```python
from build123d import *

# Parameters (mm, degrees)
CYLINDER038_R     = 0.8
CYLINDER038_DEPTH = 30
BOX040_W          = 21
BOX040_H          = 20
BOX040_DEPTH      = 18
CHAMFER_SIZE      = 8
BOX041_W          = 13
BOX041_H          = 20
BOX041_DEPTH      = 5
FILLET002033_R    = 3
BOX031_W          = 21
BOX031_H          = 20
BOX031_DEPTH      = 18
FILLET002030_R    = 3
FILLET002031_R    = 3
FILLET002032_R    = 3


with BuildPart() as obj1:
    # Cylinder038 → Cylinder038 (new body)
    with BuildSketch(Plane(origin=(42, 45, 26), x_dir=(1, 0, 0), z_dir=(0, 1, 0))):
        Circle(CYLINDER038_R)
    extrude(amount=CYLINDER038_DEPTH)


with BuildPart() as fusion024:
    # Box040 → Box040 (new body)
    with BuildSketch(Plane(origin=(40, 51.5, 10), x_dir=(1, 0, 0), z_dir=(0, 0, 1))):
        with Locations((10.5, 10)):
            Rectangle(BOX040_W, BOX040_H)
    extrude(amount=BOX040_DEPTH)

    # Chamfer
    chamfer_edges = [fusion024.edges().sort_by_distance(p)[0] for p in [
        (40, 61.5, 28),
    ]]
    chamfer(chamfer_edges, length=CHAMFER_SIZE)

    # Fusion024: union obj1
    add(obj1.part)


with BuildPart() as fillet002033:
    # Box041 → Box041 (new body)
    with BuildSketch(Plane(origin=(45, 51.5, 28), x_dir=(1, 0, 0), z_dir=(0, 0, 1))):
        with Locations((6.5, 10)):
            Rectangle(BOX041_W, BOX041_H)
    extrude(amount=BOX041_DEPTH)

    # Fillet002033
    fillet002033_edges = [fillet002033.edges().sort_by_distance(p)[0] for p in [
        (45, 51.5, 30.5),
        (45, 71.5, 30.5),
        (58, 51.5, 30.5),
        (58, 71.5, 30.5),
    ]]
    fillet(fillet002033_edges, radius=FILLET002033_R)


with BuildPart() as button:
    # Box031 → Box031 (new body)
    with BuildSketch(Plane(origin=(37, 51.5, 13), x_dir=(1, 0, 0), z_dir=(0, 0, 1))):
        with Locations((10.5, 10)):
            Rectangle(BOX031_W, BOX031_H)
    extrude(amount=BOX031_DEPTH)

    # Fillet002030
    fillet002030_edges = [button.edges().sort_by_distance(p)[0] for p in [
        (58, 51.5, 22),
        (58, 71.5, 22),
    ]]
    fillet(fillet002030_edges, radius=FILLET002030_R)

    # Fillet002031
    fillet002031_edges = [button.edges().sort_by_distance(p)[0] for p in [
        (46, 71.5, 13),
        (46, 51.5, 13),
    ]]
    fillet(fillet002031_edges, radius=FILLET002031_R)

    # Fillet002032
    fillet002032_edges = [button.edges().sort_by_distance(p)[0] for p in [
        (37, 61.5, 31),
    ]]
    fillet(fillet002032_edges, radius=FILLET002032_R)

    # Fusion025: union Fillet002033
    add(fillet002033.part)

    # Cut006: cut Fusion024
    add(fusion024.part, mode=Mode.SUBTRACT)


solid = button.part
```
The listing builds one solid part. Answer for the finished solid, in the listing's coordinates (mm). A direction names the side the tool comes from. Give positions to 0.01 mm unless a question says otherwise; leave off trailing zeros. Order: outer loops, then holes, each group sorted by start corner. A loop starts at its lowest first (then second) coordinate and runs counter-clockwise, first axis right, second up. Notation, with made-up numbers: (32.5, -19) -> (45.5, -19) arc R17 cw to (45.5, -15) -> close; hole circle Ø7 at (46.5, -35.75). An arc over 180 degrees is marked (long way). One line per item, written item: value.
1) Determine the mould class of faces 1 (the cylindrical face through (37.9, 61.64, 30.14)), 2 (the cylindrical face through (57.1, 52.36, 30.54)), 3 (the cylindrical face through (38.52, 70.6, 13.86)), 4 (the cylindrical face through (41.2, 61.4, 26)) for opening direction Z: pulls with the +Z half, pulls with the -Z half, needs draft (parallel to the pull), parting line crosses it, or undercut.
Reported:
face 1: pulls with the +Z half
face 2: needs draft
face 3: pulls with the -Z half
face 4: undercut
2) Find section B-B, the plane x = 42. Determine the outline of the cut face in (y, z).
Reported:
outline: (51.5, 22) -> (71.5, 22) -> (71.5, 25.2) -> (51.5, 25.2) -> close; (51.5, 26.8) -> (71.5, 26.8) -> (71.5, 31) -> (51.5, 31) -> close
3) Find section A-A, the plane z = 26. Determine the outline of the cut face in (x, y).
Reported:
outline: (37, 51.5) -> (41.2, 51.5) -> (41.2, 71.5) -> (37, 71.5) -> close; (42.8, 51.5) -> (46, 51.5) -> (46, 71.5) -> (42.8, 71.5) -> close
4) Find the intervals of material crossed by line 1 (Z direction, x = 54.5, y = 67.5); line 2 (X direction, y = 64.75, z = 31.75); line 3 (Z direction, x = 42, y = 62.5), in increasing order.
Reported:
line 1: z = 28 to 33
line 2: x = 45 to 58
line 3: z = 22 to 25.2, 26.8 to 31
5) Flat-ended cylindrical pins translate along their axes: P1, Ø5.5, axis at y = 60.5, z = 15.5, coming from the +X side; P2, Ø1, axis at x = 42, z = 26, coming from the -Y side; P3, Ø2.5, axis at x = 43.5, y = 65, coming from the +Z side; P4, Ø10, axis at x = 47, y = 59, coming from the -Z side. Find the tip coordinate at first contact, or state that the pin passes through.
Reported:
P1: stops at x = 40
P2: passes through
P3: stops at z = 31
P4: stops at z = 22
6) Find section D-D, the plane x = 49.25. Determine the outline of the cut face in (y, z).
Reported:
outline: (51.5, 28) -> (71.5, 28) -> (71.5, 33) -> (51.5, 33) -> close
7) Find section C-C, the plane y = 57. Determine the outline of the cut face in (x, z).
Reported:
outline: (37, 13) -> (40, 13) -> (40, 20) -> (48, 28) -> (58, 28) -> (58, 33) -> (45, 33) -> (45, 31) -> (40, 31) arc R3 ccw to (37, 28) -> close; hole circle Ø1.6 at (42, 26)
8) A tool of negligible diameter and unlimited length cuts with its end or side. For faces 5 (the cylindrical face through (45.86, 52.4, 32.01)), 6 (the cylindrical face through (45.86, 70.6, 32.01)), 7 (the flat face through (53, 62, 28)), from which of +Z, -Z, +X, -X, +Y, -Y can it reach the whole face along a straight path? Write none if from no direction.
Reported:
face 5: +Z, -X, -Y
face 6: +Z, -X, +Y
face 7: -Z, +X, +Y, -Y
